Read the model definition and answer for the solid it produces. Units are mm, in the model's axes. A direction names the side the tool comes from. Coordinates: 2 decimals unless noted, no trailing zeros. Write each loop counter-clockwise with the first axis right and the second up, starting at its lowest first coordinate (ties: lowest second). Pieces come first, ordered by that corner, then holes.
Item 1: Section C-C (z = 4.25) is taken. Give the vertices of the cut face in (x, y).
Item 2: Each of these flat-tipped pins is pushed along its axis until it touches: P1, Ø0.8, axis at y = 31, z = 2.5, coming from the -X side; P2, Ø3, axis at x = -25, y = -15.5, coming from the -Z side; P3, Ø3, axis at x = 25, y = -16, coming from the -Z side. Where does it stop, or does it pass through?
Item 3: Determine the mould class of faces 4 (the face through (25.74, 14.41, 2.46)), 5 (the face through (-13.2, -24.1, 0)), 6 (the face through (25.11, -17.96, 2.46)) for opening direction Y: released by +Y, released by -Y, zero draft, split by the parting line, or undercut.
Item 4: Straight lines are drawn through the part: probe 1 along Y at (x, z) = (0, 2.25); probe 2 along Y at (x, z) = (-1, 1.75); probe 3 along Y at (x, z) = (0, 2.75). For each, find the intervals that lie inside material, in ascending order.
Item 5: A tool of negligible diameter and unlimited length cuts with its end or side. For faces 1 (the face through (-25.6, -14.9, 2)), 2 (the face through (0.04, 30.71, 0.6)), 3 (the face through (28.141, -12.783, 2.461)), from which of +Z, -Z, +X, -X, +Y, -Y can it reach the whole face along a straight path? Write none if from no direction.
Item 6: Section B-B (y = 0) is taken. Give the vertices of the cut face in (x, z).
from build123d import *

# Parameters (mm, degrees)
F0_R     = 29.5
F0_R_2   = 25.25
F1_DEPTH = 5
F3_W     = 6
F3_H     = 5
F4_DEPTH = 5
F5_R     = 3
F6_W     = 6
F6_H     = 0.7910079116
F7_DEPTH = 2
F8_R     = 1.99999


# Not quite as in the source:
# - a fillet or chamfer is up to 0.001 mm smaller than in the source, because OpenCascade refuses the exact size
# - a feature of the source that left no trace in its solid (it failed there, or was rolled back) is left out


with BuildPart() as f1:
    # F0 (on Top) → F1 (new body)
    with BuildSketch(Plane.XY):
        Circle(F0_R)
        Circle(F0_R_2, mode=Mode.SUBTRACT)
    extrude(amount=F1_DEPTH)

    # F3 (on Top) → F4 (join)
    with BuildSketch(Plane.XY):
        with Locations((0, 29.6380690932)):
            Rectangle(F3_W, F3_H)
        Polygon((-29.3323842633, -13.4709583353), (-26.3323842633, -18.667110758), (-22.0022572444, -16.167110758), (-25.0022572444, -10.9709583353), align=None)
        Polygon((26.3323842633, -18.667110758), (29.3323842633, -13.4709583353), (25.0022572444, -10.9709583353), (22.0022572444, -16.167110758), align=None)
    extrude(amount=F4_DEPTH)

    # F5
    f5_edges = [f1.edges().sort_by_distance(p)[0] for p in [
        (0, 32.138069, 5),
        (-27.832384, -16.069035, 5),
        (27.832384, -16.069035, 5),
    ]]
    fillet(f5_edges, radius=F5_R)

    # F6 (on face) → F7 (cut)
    with BuildSketch(Plane(origin=(0, 0, 0), x_dir=(1, 0, 0), z_dir=(0, 0, -1))):
        with Locations((0, -29.7425651374)):
            Rectangle(F6_W, F6_H)
        Polygon((24.6003334557, 17.667110758), (23.9153005097, 17.2716068022), (26.9153005097, 12.0754543795), (27.6003334557, 12.4709583353), align=None)
        Polygon((-27.6003334557, 12.4709583353), (-26.9153005097, 12.0754543795), (-23.9153005097, 17.2716068022), (-24.6003334557, 17.667110758), align=None)
    extrude(amount=-F7_DEPTH, mode=Mode.SUBTRACT)

    # F8 (radius 2 in the source; OpenCascade refuses exactly that, so slightly less here)
    f8_edges = [f1.edges().sort_by_distance(p)[0] for p in [
        (0, 29.347061, 0),
        (0, 30.138069, 0),
        (26.100333, -15.069035, 0),
        (25.415301, -14.673531, 0),
        (-25.415301, -14.673531, 0),
        (-26.100333, -15.069035, 0),
        (-25.25, 0, 0),
        (-25.25, 0, 5),
    ]]
    fillet(f8_edges, radius=F8_R)


solid = f1.part
Established:
1. outline: (-28.45, -12.96) - (-25.45, -18.16) - (-23.92, -17.27) arc R29.5 ccw to (23.92, -17.27) - (25.45, -18.16) - (28.45, -12.96) - (26.92, -12.08) arc R29.5 ccw to (3, 29.35) - (3, 31.12) - (-3, 31.12) - (-3, 29.35) arc R29.5 ccw to (-26.92, -12.08) - close; hole circle Ø51.38 at (0, 0)
2. P1: stops at x = -3
2. P2: stops at z = 0.08
2. P3: stops at z = 0.17
3. face 4: undercut
3. face 5: zero draft
3. face 6: released by -Y
4. probe 1: y = -29.5 to -25.25, 25.25 to 32.13
4. probe 2: y = -29.48 to -25.25, 25.25 to 29.33, 30.15 to 32.14
4. probe 3: y = -29.5 to -25.25, 25.25 to 32.04
5. face 1: -Z
5. face 2: -Z, +X, -X
5. face 3: +Z, -Z, +X
6. outline: (-29.5, 0) - (-27.25, 0) arc R2 ccw to (-25.25, 2) - (-25.25, 3) arc R2 ccw to (-27.25, 5) - (-29.5, 5) - close; (25.25, 2) arc R2 ccw to (27.25, 0) - (29.5, 0) - (29.5, 5) - (27.25, 5) arc R2 ccw to (25.25, 3) - close
